Read the model definition and answer for the solid it produces. Units are mm, in the model's axes. Coordinates: 2 decimals unless noted, no trailing zeros. Loops run counter-clockwise (first coordinate to the right, second up) from the corner with the lowest first, then second, coordinate; pieces in that order, holes last. Notation, with made-up numbers: M 41,-15.5 L 52,-15.5 A23 ccw 52,0.5 Z; hole C -29,7 d3. An arc over 180 degrees is marked long. One line per item, written item: value. Start each with the question number.
```python
from build123d import *

# Parameters (mm, degrees)
BASE_FLANGE1_DEPTH = 139.7


# Sheet-metal steps are written as plain solids
with BuildPart() as part:
    # Sketch1 → Base-Flange1 (new body)
    with BuildSketch(Plane.XY):
        with BuildLine():
            ThreePointArc((78.58125, 136.106717522), (136.106717522, 78.58125), (157.1625, 0))
            ThreePointArc((157.1625, 0), (111.130669498, -111.130669498), (0, -157.1625))
            Line((0, -157.1625), (0, -158.75))
            ThreePointArc((0, -158.75), (112.253201513, -112.253201513), (158.75, 0))
            ThreePointArc((158.75, 0), (137.481532851, 79.375), (79.375, 137.481532851))
            Line((79.375, 137.481532851), (78.58125, 136.106717522))
        make_face()
    extrude(amount=BASE_FLANGE1_DEPTH)


solid = part.part
```
1) Flat-ended cylindrical pins translate along their axes: pin 1 (3 mm diameter, centred on y = -68, z = 53.5, fed in from +X); pin 2 (3 mm diameter, centred on y = -89, z = 85.5, fed in from +X); pin 3 (2 mm diameter, centred on y = 86.5, z = 116.5, fed in from -X). Find the tip coordinate at first contact, or state that the pin passes through.
2) Section C-C (y = 103.5) is taken. Determine the outline of the cut face in (x, z).
3) Consider line 1 along X through (y, z) = (-2, 27); line 2 along Y through (x, z) = (92.5, 55.5); line 3 along Y through (x, z) = (124.5, 74). Determine where each line is inside the solid, lowest interval first.
4) Section A-A (x = 126.5) is taken. Determine the outline of the cut face in (y, z).
5) Section D-D (x = 32.5) is taken. Determine the outline of the cut face in (y, z).
Results found:
1. pin 1: stops at x = 144.15
1. pin 2: stops at x = 132.46
1. pin 3: stops at x = 130.55
2. outline: M 118.27,0 L 120.37,0 L 120.37,139.7 L 118.27,139.7 Z
3. line 1: x = 157.15 to 158.74
3. line 2: y = -129.02 to -127.06, 127.06 to 129.02
3. line 3: y = -98.5 to -95.92, 95.92 to 98.5
4. outline: M -95.91,0 L -93.26,0 L -93.26,139.7 L -95.91,139.7 Z; M 93.26,0 L 95.91,0 L 95.91,139.7 L 93.26,139.7 Z
5. outline: M -155.39,0 L -153.77,0 L -153.77,139.7 L -155.39,139.7 Z
